The model under review builds one solid part; all positions refer to its coordinate system, in mm. Coordinates: 2 decimals unless noted, no trailing zeros. Order: outer loops, then holes, each group sorted by start corner. A loop starts at its lowest first (then second) coordinate and runs counter-clockwise, first axis right, second up.
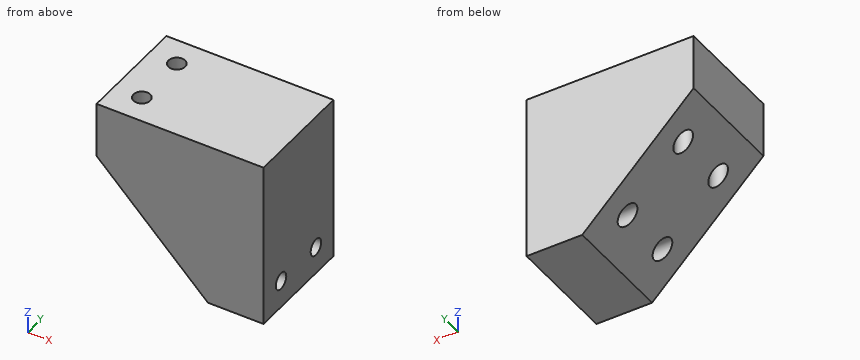
```python
from build123d import *

# Parameters (mm, degrees)
BOSS_EXTRUDE1_DEPTH = 6.35
SKETCH2_R           = 0.9525
CUT_EXTRUDE1_DEPTH  = 23.455171572
SKETCH3_R           = 0.9525
CUT_EXTRUDE2_DEPTH  = 23.234798889


with BuildPart() as part:
    # Sketch1 → Boss-Extrude1 (new, symmetric)
    with BuildSketch(Plane(origin=(0, 0, 0), x_dir=(1, 0, 0), z_dir=(0, 1, 0))):
        Polygon((-9.547841727, -2.649640288), (3.152158273, 10.050359712), (9.502158273, 10.050359712), (9.502158273, -8.999640288), (-9.547841727, -8.999640288), align=None)
    extrude(amount=BOSS_EXTRUDE1_DEPTH, both=True)

    # Sketch2 → Cut-Extrude1 (cut, through all)
    with BuildSketch(Plane(origin=(9.502158273, 0, 0), x_dir=(0, 0, -1), z_dir=(1, 0, 0))):
        with Locations((6.875359712, 3.175)):
            Circle(SKETCH2_R)
        with Locations((6.875359712, -3.175)):
            Circle(SKETCH2_R)
    extrude(amount=-CUT_EXTRUDE1_DEPTH, mode=Mode.SUBTRACT)

    # Sketch3 → Cut-Extrude2 (cut, through all)
    with BuildSketch(Plane.XY.offset(8.999640288)):
        with Locations((-6.372841727, 3.175)):
            Circle(SKETCH3_R)
        with Locations((-6.372841727, -3.175)):
            Circle(SKETCH3_R)
    extrude(amount=-CUT_EXTRUDE2_DEPTH, mode=Mode.SUBTRACT)


solid = part.part
```
(1) We need section C-C, the plane z = 4.5. Count the separate pieces of the cut face and the enclosed holes in it, and give its area (3 significant figures).
A:
separate pieces: 1
enclosed holes: 2
area: 236 mm2
(2) We need section A-A, the plane y = -2.75. Write out the cut boundary in (x, z), and give its area (3 significant figures).
A:
outline: (-9.55, 2.65) - (-7.23, 0.33) - (-7.23, 9) - (-9.55, 9) - close; (-5.52, -1.38) - (-0.88, -6.02) - (9.5, -6.02) - (9.5, 9) - (-5.52, 9) - close; (0.83, -7.73) - (3.15, -10.05) - (9.5, -10.05) - (9.5, -7.73) - close
area: 250 mm2
(3) We need section B-B, the plane y = -0.5. Write out the cut boundary in (x, z).
A:
outline: (-9.55, 2.65) - (3.15, -10.05) - (9.5, -10.05) - (9.5, 9) - (-9.55, 9) - close
(4) Wall thickness on probe 1 along Y at (x, z) = (3, -7.25); probe 2 along Y at (x, z) = (-6.25, 3.75); probe 3 along Z at (x, y) = (8, 2.5): over which ranges is each line inside the solid? List them lowest first.
A:
probe 1: y = -6.35 to -4.05, -2.3 to 2.3, 4.05 to 6.35
probe 2: y = -6.35 to -4.12, -2.23 to 2.23, 4.12 to 6.35
probe 3: z = -10.05 to -7.55, -6.2 to 9
(5) For pin 1 Ø2.5 at (y, z) = (-3.18, -6.88) entering from +X; pin 2 Ø2 at (y, z) = (2.5, -5.5) entering from -X, all flat-tipped, find the tip position at first contact; note any pin that passes through.
A:
pin 1: stops at x = 9.5
pin 2: stops at x = -2.4
